Input: part model. Units: mm. Frame: model coordinates. Round coordinates to 2 decimals unless told otherwise and drop trailing zeros. Loops run counter-clockwise (first coordinate to the right, second up) from the corner with the lowest first, then second, coordinate; pieces in that order, holes last. Notation, with made-up numbers: M 23,34 L 64,34 A13 cw 64,59 Z; hole C 87,-13 d10. An arc over 180 degrees is marked long. Return JSON: item names as keys, results as strings. Group by question number.
1) Contact query for flat-ended pins moving along their axis: P1, Ø3, axis at y = 358, z = -4.5, coming from the -X side; P2, Ø1, axis at y = 60.5, z = 1.5, coming from the -X side (3 decimals); P3, Ø1.5, axis at x = 0, z = -0.5, coming from the +Y side. Output: stop coordinate, or through.
2) Section A-A (y = 117). Output: boundary loops of the cut face in (x, z), plus the area to 3 significant figures.
3) Material intervals for line 1 (Z direction, x = 0, y = 396.25); line 2 (X direction, y = 388.5, z = 0); line 3 (Y direction, x = -0.25, z = 1), sorted ascending. Write a range as from..to.
from build123d import *

# Parameters (mm, degrees)
BOSS_EXTRUDE1_DEPTH = 406.4
SKETCH2_R           = 2.54
CUT_EXTRUDE1_DEPTH  = 25.4
SKETCH3_R           = 6.35
BOSS_EXTRUDE2_DEPTH = 0.254


with BuildPart() as part:
    # Sketch1 → Boss-Extrude1 (new body)
    with BuildSketch(Plane(origin=(0, 0, 0), x_dir=(1, 0, 0), z_dir=(0, 1, 0))):
        Polygon((7.332348419, 0), (3.666174209, 6.35), (-3.666174209, 6.35), (-7.332348419, 0), (-3.666174209, -6.35), (3.666174209, -6.35), align=None)
    extrude(amount=BOSS_EXTRUDE1_DEPTH)

    # Sketch2 → Cut-Extrude1 (cut)
    with BuildSketch(Plane(origin=(0, 406.4, 0), x_dir=(1, 0, 0), z_dir=(0, 1, 0))):
        Circle(SKETCH2_R)
    extrude(amount=-CUT_EXTRUDE1_DEPTH, mode=Mode.SUBTRACT)

    # Sketch3 → Boss-Extrude2 (add)
    with BuildSketch(Plane.XZ):
        Circle(SKETCH3_R)
    extrude(amount=BOSS_EXTRUDE2_DEPTH)


solid = part.part
Returned:
{
 "1": {"P1": "stops at x = -5.6", "P2": "stops at x = -6.755", "P3": "stops at y = 381"},
 "2": {"outline": "M -7.33,0 L -3.67,-6.35 L 3.67,-6.35 L 7.33,0 L 3.67,6.35 L -3.67,6.35 Z", "area": "140 mm^2"},
 "3": {"line 1": "z = -6.35..-2.54, 2.54..6.35", "line 2": "x = -7.33..-2.54, 2.54..7.33", "line 3": "y = -0.25..381"}
}
